Geometry check sheet. Reference: the model listing, model coordinates, mm. Give positions to 0.01 mm unless a question says otherwise; leave off trailing zeros. Loops run counter-clockwise (first coordinate to the right, second up) from the corner with the lowest first, then second, coordinate; pieces in that order, holes last. Notation, with made-up numbers: (-11, -36.5) -> (8, -36.5) arc R25 cw to (8, -2.5) -> close; hole circle Ø8 at (24.25, 70.25). An arc over 180 degrees is marked (long way). Write each question's results on one line, items separated by ' | '. Start each with the question number.
1) Sectioned sample at A-A on x = 0. Record the cut outline in (y, z).
2) Depth check by flat-ended pin: pin 1 (2 mm diameter, centred on x = 4, z = 3, fed in from +Y); pin 2 (1 mm diameter, centred on y = 0.5, z = 2.5, fed in from -X); pin 3 (1 mm diameter, centred on y = -1.5, z = 3.5, fed in from +X). Enter the tip coordinate at first touch or a pass-through.
3) Sectioned sample at C-C on z = 2.45. Record the cut outline in (x, y).
4) Draft check along Y on faces 1 (the face through (-1.172, 8.923, 2.23)), 2 (the face through (-6, 0, 2)), 3 (the face through (6, 3, 4)). Enter one of: pulls with the +Y half, pulls with the -Y half, needs draft (parallel to the pull), parting line crosses it, or undercut.
5) Scan lines: line 1 (Y direction, x = 0, z = 1.5); line 2 (Y direction, x = 4.25, z = 3.8); line 3 (X direction, y = -3, z = 2.6). Record each from-to range of solid material in increasing order. Write a range as from..to.
```python
from build123d import *

# Parameters (mm, degrees)
SKETCH_1_R      = 9
SKETCH_1_R_2    = 6
EXTRUDE_1_DEPTH = 4
SKETCH_2_R      = 9.75
SKETCH_2_R_2    = 9
EXTRUDE_2_DEPTH = 0.8
CHAMFER_1_SIZE  = 0.3


with BuildPart() as part:
    # 草图1 → 凸台-拉伸1 (new body)
    with BuildSketch(Plane.XY):
        Circle(SKETCH_1_R)
        Circle(SKETCH_1_R_2, mode=Mode.SUBTRACT)
    extrude(amount=EXTRUDE_1_DEPTH)

    # 草图2 → 凸台-拉伸2 (add)
    with BuildSketch(Plane(origin=(0, 0, 0), x_dir=(-1, 0, 0), z_dir=(0, 0, -1))):
        Circle(SKETCH_2_R)
        Circle(SKETCH_2_R_2, mode=Mode.SUBTRACT)
    extrude(amount=-EXTRUDE_2_DEPTH)

    # 倒角1
    chamfer_1_edges = [part.edges().sort_by_distance(p)[0] for p in [
        (9.75, 0, 0.8),
        (9.75, 0, 0),
        (-9, 0, 4),
        (-6, 0, 0),
        (-6, 0, 4),
    ]]
    chamfer(chamfer_1_edges, length=CHAMFER_1_SIZE)


solid = part.part
```
Result:
1) outline: (-9.75, 0.3) -> (-9.45, 0) -> (-6.3, 0) -> (-6, 0.3) -> (-6, 3.7) -> (-6.3, 4) -> (-8.7, 4) -> (-9, 3.7) -> (-9, 0.8) -> (-9.45, 0.8) -> (-9.75, 0.5) -> close; (6, 0.3) -> (6.3, 0) -> (9.45, 0) -> (9.75, 0.3) -> (9.75, 0.5) -> (9.45, 0.8) -> (9, 0.8) -> (9, 3.7) -> (8.7, 4) -> (6.3, 4) -> (6, 3.7) -> close
2) pin 1: y = 8.49 | pin 2: x = -9 | pin 3: x = 8.94
3) outline: circle Ø18 at (0, 0); hole circle Ø12 at (0, 0)
4) face 1: parting line crosses it | face 2: undercut | face 3: needs draft
5) line 1: -9..-6, 6..9 | line 2: -7.82..-4.38, 4.38..7.82 | line 3: -8.49..-5.2, 5.2..8.49
